from build123d import *

# Parameters (mm, degrees)
SKETCH_1_R          = 6
SKETCH_1_R_2        = 3
EXTRUDE_1_DEPTH     = 3.2
SKETCH_2_R          = 6.8
EXTRUDE_2_DEPTH     = 0.8
SKETCH_3_R          = 3
CUT_EXTRUDE_1_DEPTH = 0.8


with BuildPart() as part:
    # 草图1 → 凸台-拉伸1 (new body)
    with BuildSketch(Plane.XY):
        Circle(SKETCH_1_R)
        Circle(SKETCH_1_R_2, mode=Mode.SUBTRACT)
    extrude(amount=EXTRUDE_1_DEPTH)

    # 草图2 → 凸台-拉伸2 (add)
    with BuildSketch(Plane.XY.offset(3.2)):
        Circle(SKETCH_2_R)
    extrude(amount=EXTRUDE_2_DEPTH)

    # 草图3 → 切除-拉伸1 (cut)
    with BuildSketch(Plane(origin=(0, 0, 3.2), x_dir=(-1, 0, 0), z_dir=(0, 0, -1))):
        Circle(SKETCH_3_R)
    extrude(amount=-CUT_EXTRUDE_1_DEPTH, mode=Mode.SUBTRACT)


solid = part.part
Verification items for the finished model (mm, model axes). A direction names the side the tool comes from. Coordinates: 2 decimals unless noted, no trailing zeros. Order: outer loops, then holes, each group sorted by start corner. A loop starts at its lowest first (then second) coordinate and runs counter-clockwise, first axis right, second up. Notation, with made-up numbers: M -18.5,24.25 L 13.5,24.25 A25 cw 13.5,48.25 Z; hole C -2.75,-28.75 d11. An arc over 180 degrees is marked long. One line per item, written item: value. Start each with the question number.
Item 1: Sectioned sample at A-A (y = 0). Enter the section's corners in (x, z), then the cut area to 3 significant figures.
Item 2: Sectioned sample at C-C (z = 2.65). Enter the section's corners in (x, y), then the cut area to 3 significant figures.
Item 3: Access from +Z, -Z, +X, -X, +Y, -Y to the whole of each face (thin tool, end or side, straight path). Record for faces 1 (the flat face through (4, -5, 3.2)), 2 (the cylindrical face through (-1.47, -6.64, 3.59)).
Item 4: Sectioned sample at D-D (x = 4.25). Enter the section's corners in (y, z).
Item 5: Gauge pin test, flat ends, axial feed: pin 1 (1 mm diameter, centred on y = -2.5, z = 2.5, fed in from +X); pin 2 (1 mm diameter, centred on y = 5, z = 2, fed in from -X). Record the tip position at first contact, or that the pin passes through.
Item 6: Scan lines: probe 1 along Y at (x, z) = (0, 1.3); probe 2 along Y at (x, z) = (0, 3.65); probe 3 along X at (y, z) = (-2.5, 2.75). Record each from-to range of solid material in increasing order.
Conclusion:
1. outline: M -6.8,3.2 L -6,3.2 L -6,0 L -3,0 L -3,4 L -6.8,4 Z; M 3,0 L 6,0 L 6,3.2 L 6.8,3.2 L 6.8,4 L 3,4 Z
1. area: 25.3 mm^2
2. outline: C 0,0 d12; hole C 0,0 d6
2. area: 84.8 mm^2
3. face 1: -Z
3. face 2: +Z, -Z
4. outline: M -5.31,3.2 L -4.24,3.2 L -4.24,0 L 4.24,0 L 4.24,3.2 L 5.31,3.2 L 5.31,4 L -5.31,4 Z
5. pin 1: stops at x = 5.66
5. pin 2: stops at x = -3.97
6. probe 1: y = -6 to -3, 3 to 6
6. probe 2: y = -6.8 to -3, 3 to 6.8
6. probe 3: x = -5.45 to -1.66, 1.66 to 5.45
